Check sheet for the modelled part. Datum: model origin and axes. Units: mm. A direction names the side the tool comes from. Round coordinates to 2 decimals unless told otherwise and drop trailing zeros. Write each loop counter-clockwise with the first axis right and the second up, starting at its lowest first coordinate (ties: lowest second). Pieces come first, ordered by that corner, then holes. Notation, with made-up numbers: (27.5, 9.25) -> (86.5, 9.25) arc R27 cw to (86.5, 45.25) -> close; hole circle Ø1 at (21.5, 82). An arc over 180 degrees is marked (long way). Put each result on its own line as item: value. Start each with the question number.
Autodesk Inventor part; units mm, degrees
ref_plane "YZ Plane" through (0, 0, 0) normal (1, 0, 0) x (0, 1, 0)
ref_plane "XZ Plane" through (0, 0, 0) normal (0, 1, 0) x (-1, 0, 0)
ref_plane "XY Plane" through (0, 0, 0) normal (0, 0, 1) x (1, 0, 0)
sketch "Szkic1" plane through (0, 0, 0) normal (0, 0, 1) x (1, 0, 0)
  line L0 (-10, 4) -> (10, 4)
  line L1 (10, 4) -> (10, -4)
  line L2 (10, -4) -> (-10, -4)
  line L3 (-10, -4) -> (-10, 4)
  line L4 (-10, 4) -> (10, -4) construction
  line L5 (10, 4) -> (-10, -4) construction
  point P0 (0, 0)
  dimension "d0" = 8
  dimension "d1" = 20
extrude "Wyciągnięcie proste1" add sketch "Szkic1" along normal blind 3
sketch "Szkic2" plane through (0, 0, 3) normal (0, 0, 1) x (1, 0, 0)
  line L0 (-10, 4) -> (-10, -4)
  point P0 (0, 0)
  point P1 (-4, 0)
  point P2 (4, 0)
  dimension "d6" = 8
  dimension "d7" = 6
hole "Otwór1" at (-4, 0, 3) at (4, 0, 3) direction (0, 0, -1) diameter 4.134 depth 7 tip angle 118 countersink diameter 7 countersink angle 90
sketch "Szkic3" plane through (0, 0, 3) normal (0, 0, 1) x (1, 0, 0)
  line L0 (10, 4) -> (-10, 4)
  line L1 (-10, -4) -> (10, -4)
  line L2 (10, 4) -> (7.6326, 4)
  line L3 (7.6326, 4) -> (7.6326, -4)
  line L4 (7.6326, -4) -> (10, -4)
  line L5 (10, -4) -> (10, 4)
  point P0 (0, 0)
  point P1 (10, -4)
extrude "Wyciągnięcie proste2" add sketch "Szkic3" along normal blind 1
sketch "Szkic4" plane through (0, 0, 4) normal (0, 0, 1) x (1, 0, 0)
  line L0 (10, -4) -> (10, 4)
  line L1 (10, -4) -> (7.633, -4)
  line L2 (7.633, -4) -> (7.633, 26)
  line L3 (7.633, 26) -> (10, 26)
  line L4 (10, 26) -> (10, -4)
  point P0 (0, 0)
  dimension "d17" = 2.367
  dimension "d18" = 30
extrude "Wyciągnięcie proste3" add sketch "Szkic4" along normal blind 20
properties part number "chwyt"
1. Access from +Z, -Z, +X, -X, +Y, -Y to the whole of each face (thin tool, end or side, straight path). Record for faces 1 (the flat face through (-10, 0, 1)), 2 (the flat face through (9, 15, 4)), 3 (the flat face through (7.633, 0.1, 3.5)).
2. Section check D-D, the plane y = 17. Enter the section's corners in (x, z), then the cut area to 3 significant figures.
3. Section check A-A, the plane x = 4. Enter the section's corners in (y, z), then the cut area to 3 significant figures.
4. Material ranges on L1, parallel to X at y = 0, z = 1; L2, parallel to X at y = 1, z = 1.75; L3, parallel to Y at x = -4, z = 1, recorded low to high. Write a range as [from, to].
5. Section check B-B, the plane y = 0. Give the number of separate pieces and of enclosed holes in the cut face, then the cut area to 3 significant figures.
6. Draft check along X on faces 4 (the conical face through (4.1, 2.2, 1.7)), 5 (the flat face through (7.633, 11, 14)), 6 (the flat face through (9, 26, 14)). Enter one of: released by +X, released by -X, zero draft, split by the parting line, or undercut.
7. Gauge pin test, flat ends, axial feed: P1, Ø0.7, axis at x = 8.5, y = 11.5, coming from the -Z side; P2, Ø4.5, axis at x = 0.5, z = 3, coming from the +Y side; P3, Ø5.5, axis at x = -4, y = 0, coming from the -Z side; P4, Ø0.5, axis at y = -0.5, z = 3.5, coming from the -X side. Record the tip position at first contact, or that the pin passes through.
8. Section check C-C, the plane z = 5.25. Enter the section's corners in (x, y), then the cut area to 3 significant figures.
Reply:
1. face 1: +Z, -Z, -X, +Y, -Y
1. face 2: -Z, +X, -X, +Y
1. face 3: +Z, -X, +Y, -Y
2. outline: (7.63, 4) -> (10, 4) -> (10, 24) -> (7.63, 24) -> close
2. area: 47.3 mm2
3. outline: (-4, 0) -> (-2.07, 0) -> (-2.07, 1.57) -> (-3.5, 3) -> (-4, 3) -> close; (2.07, 0) -> (4, 0) -> (4, 3) -> (3.5, 3) -> (2.07, 1.57) -> close
3. area: 9.54 mm2
4. L1: x = [-10, -6.07], [-1.93, 1.93], [6.07, 10]
4. L2: x = [-10, -6.02], [-1.98, 1.98], [6.02, 10]
4. L3: y = [-4, -2.07], [2.07, 4]
5. separate pieces: 3
5. enclosed holes: 0
5. area: 80.8 mm2
6. face 4: undercut
6. face 5: released by -X
6. face 6: zero draft
7. P1: stops at z = 4
7. P2: stops at y = 4
7. P3: stops at z = 0
7. P4: stops at x = 7.63
8. outline: (7.63, -4) -> (10, -4) -> (10, 26) -> (7.63, 26) -> close
8. area: 71.0 mm2
